Can you work these out from the drawing? Everything is in mm from the part's minimum corner. A direction names the side the tool comes from. Give positions to 0.01 mm unless a question says otherwise; leave off trailing zeros. Write each loop counter-clockwise with the first axis right and the second up, starting at its lowest first coordinate (ties: lowest second). Pieces come first, ordered by that corner, then holes. Notation, with made-up numbers: (68, -22) - (106, -22) arc R34 ccw to (106, 16) - close; hole circle Ø3 at (3.25, -39.75). An arc over 180 degrees is marked (long way). Write each question's results on one line, items separated by ' | '. Start each with the question number.
Item 1: We'd pull the mould along X, two halves only. Please class the marked faces 4, 5 and 6: +X half, -X half, draft (parallel to the pull), parting line (faces both ways), or undercut.
Item 2: Suppose I cut it at B-B on z = 92.5. List the corners of the cut face in (x, y) for me (3 decimals), then the cut area to 3 significant figures.
Item 3: Which directions (+Z, -Z, +X, -X, +Y, -Y) give clear straight access to the entire face, cutting with the end or side of a thin tool? Please do the marked faces 1, 2 and 3.
Item 4: Suppose I cut it at D-D on z = 17.5. List the corners of the cut face in (x, y) for me (3 decimals).
Item 5: Suppose I cut it at A-A on y = 12.7. List the corners of the cut face in (x, z) for me (3 decimals).
Item 6: Please list where these lines run through material, in increasing order: line 1 along X through (y, z) = (3.5, 127); line 2 along Z through (x, y) = (57, 23.5) (3 decimals); line 3 along Z through (x, y) = (31.5, 2) (3 decimals).
Item 7: Suppose I cut it at C-C on x = 33.5. List the corners of the cut face in (y, z) for me (3 decimals).
Item 8: Will these pins go through, and if not, where does the flat tip stop? P1, Ø14, axis at y = 14, z = 106, coming from the +X side (3 decimals); P2, Ø4, axis at y = 5.5, z = 46, coming from the +X side; P3, Ø1, axis at x = 27.5, y = 8, coming from the -Z side.
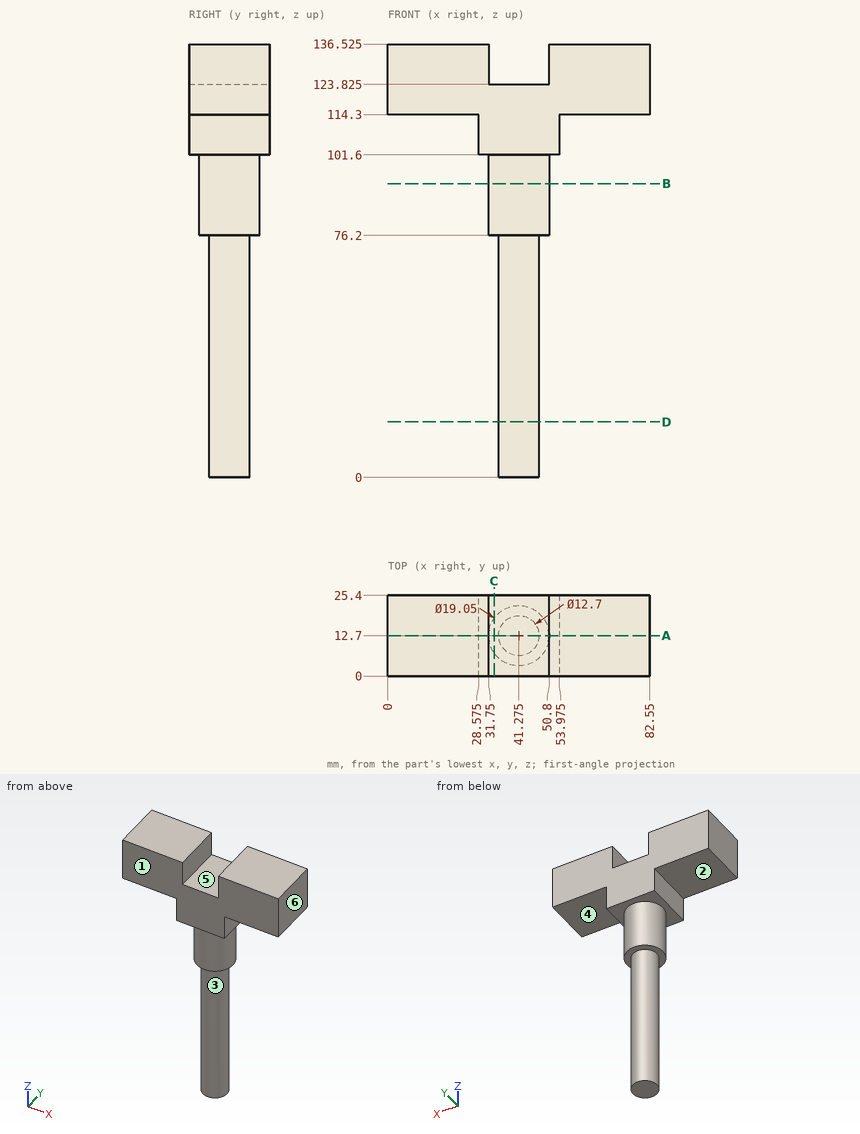
Checked values:
1) face 4: draft | face 5: undercut | face 6: +X half
2) outline: circle Ø19.05 at (41.275, 12.7) | area: 285 mm^2
3) face 1: +Z, -Z, +X, -X, -Y | face 2: -Z, -X, +Y, -Y | face 3: -Z
4) outline: circle Ø12.7 at (41.275, 12.7)
5) outline: (0, 114.3) - (28.575, 114.3) - (28.575, 101.6) - (31.75, 101.6) - (31.75, 76.2) - (34.925, 76.2) - (34.925, 0) - (47.625, 0) - (47.625, 76.2) - (50.8, 76.2) - (50.8, 101.6) - (53.975, 101.6) - (53.975, 114.3) - (82.55, 114.3) - (82.55, 136.525) - (50.8, 136.525) - (50.8, 123.825) - (31.75, 123.825) - (31.75, 136.525) - (0, 136.525) - close
6) line 1: x = 0 to 31.75, 50.8 to 82.55 | line 2: z = 114.3 to 136.525 | line 3: z = 101.6 to 136.525
7) outline: (0, 101.6) - (7.198, 101.6) - (7.198, 76.2) - (18.202, 76.2) - (18.202, 101.6) - (25.4, 101.6) - (25.4, 123.825) - (0, 123.825) - close
8) P1: stops at x = 53.975 | P2: stops at x = 44.92 | P3: stops at z = 114.3
